The figure shows three views and two pictorial views of one solid part (mm, origin at its lowest corner). Answer the questions. A direction names the side the tool comes from. Coordinates: 2 decimals unless noted, no trailing zeros. Order: outer loops, then holes, each group sorted by start corner. A loop starts at its lowest first (then second) coordinate and runs counter-clockwise, first axis right, second up. Notation, with made-up numbers: (24.5, -20) -> (29.5, -20) arc R13 ccw to (29.5, -14) -> close; hole circle Ø4 at (24.25, 36.5). An arc over 180 degrees is marked (long way). Write item = value, one per line.
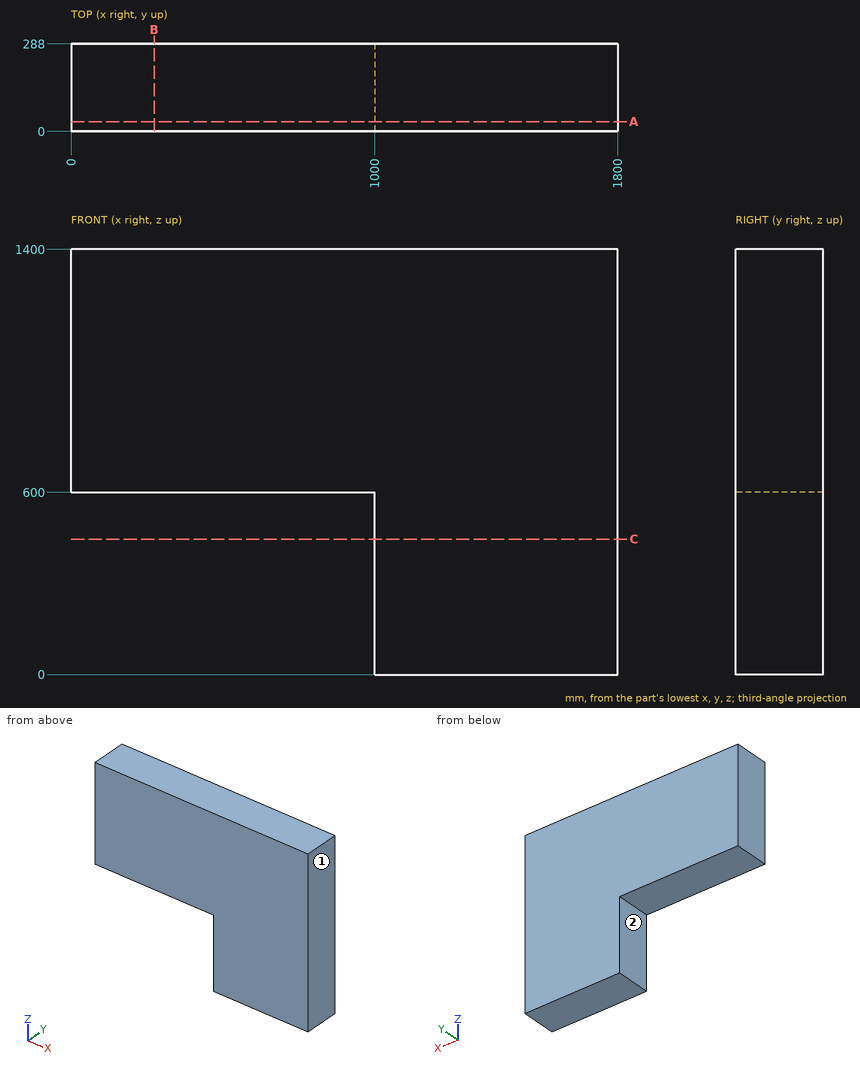
Q1. Section B-B, the plane x = 274 is taken. Give the vertices of the cut face in (y, z).
The answers:
outline = (0, 600) -> (288, 600) -> (288, 1400) -> (0, 1400) -> close
Q2. A tool of negligible diameter and unlimited length cuts with its end or side. For the marked faces 1 and 2, from which of +Z, -Z, +X, -X, +Y, -Y can it reach the whole face along a straight path? Write none if from no direction.
The answers:
face_1 = +Z, -Z, +X, +Y, -Y
face_2 = -Z, -X, +Y, -Y
Q3. Section C-C, the plane z = 446 is taken. Give the vertices of the cut face in (x, y), plus the area to 3 significant figures.
The answers:
outline = (1000, 0) -> (1800, 0) -> (1800, 288) -> (1000, 288) -> close
area = 230,000 mm2
Q4. Find the intervals of material crossed by line 1 along Z through (x, y) = (361.5, 102); line 2 along X through (y, z) = (165, 423), in increasing order.
The answers:
line_1 = 600 to 1400
line_2 = 1000 to 1800
Q5. Section A-A, the plane y = 32 is taken. Give the vertices of the cut face in (x, z), plus the area to 3 significant figures.
The answers:
outline = (0, 600) -> (1000, 600) -> (1000, 0) -> (1800, 0) -> (1800, 1400) -> (0, 1400) -> close
area = 1,920,000 mm2
